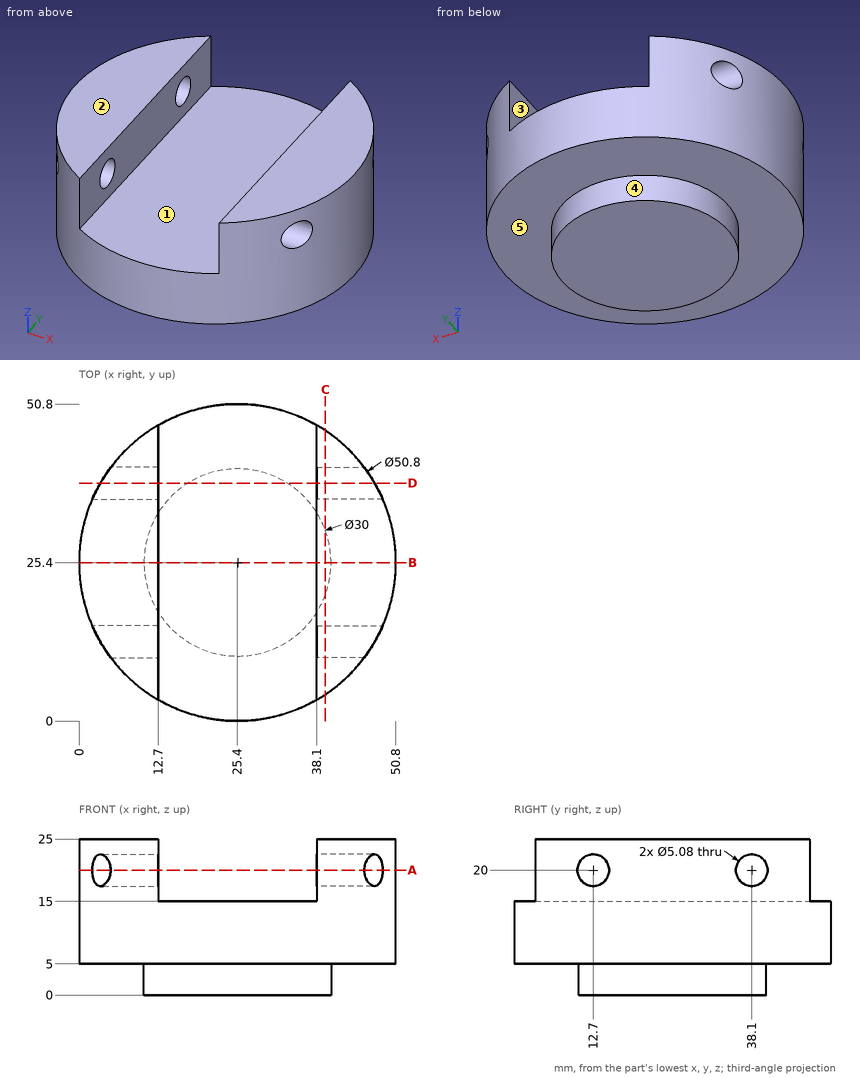
The figure shows three views and two pictorial views of one solid part (mm, origin at its lowest corner). Answer the questions. A direction names the side the tool comes from. Round coordinates to 2 decimals unless told otherwise and drop trailing zeros. Write each loop counter-clockwise with the first axis right and the second up, starting at its lowest first coordinate (ties: lowest second). Pieces come first, ordered by that corner, then holes. Notation, with made-up numbers: (34, 38) -> (40, 38) arc R22 cw to (40, 53) -> close; hole circle Ø5 at (-7.5, -11.5). An arc over 180 degrees is marked (long way). Write each question's results on one line, items separated by ' | '.
Q1. Section D-D, the plane y = 38.1 is taken. Write down the section's boundary in (x, z), then the cut area to 3 significant figures.
Data:
outline: (3.4, 5) -> (17.42, 5) -> (17.42, 0) -> (33.38, 0) -> (33.38, 5) -> (47.4, 5) -> (47.4, 17.46) -> (38.1, 17.46) -> (38.1, 15) -> (12.7, 15) -> (12.7, 17.46) -> (3.4, 17.46) -> close; (3.4, 22.54) -> (12.7, 22.54) -> (12.7, 25) -> (3.4, 25) -> close; (38.1, 22.54) -> (47.4, 22.54) -> (47.4, 25) -> (38.1, 25) -> close | area: 611 mm^2
Q2. Flat-ended cylindrical pins translate along their axes: P1, Ø12, axis at x = 28.5, y = 6, coming from the +Z side; P2, Ø8, axis at y = 38.1, z = 20, coming from the +X side; P3, Ø5, axis at x = 8.5, y = 38.5, coming from the -Z side. Find the tip coordinate at first contact, or state that the pin passes through.
Data:
P1: z = 15 | P2: x = 49.26 | P3: z = 5
Q3. Straight lines are drawn through the part: line 1 along Z through (x, y) = (42.5, 12.7); line 2 along Y through (x, z) = (7.25, 20); line 3 along Y through (x, z) = (42.75, 20). For each, find the intervals that lie inside material, in ascending order. Write a range as [from, to].
Data:
line 1: [5, 17.46], [22.54, 25] | line 2: [7.63, 10.16], [15.24, 35.56], [40.64, 43.17] | line 3: [6.85, 10.16], [15.24, 35.56], [40.64, 43.95]
Q4. Determine the mould class of the marked faces 3, 4 and 5 for opening direction X: released by +X, released by -X, zero draft, split by the parting line, or undercut.
Data:
face 3: undercut | face 4: split by the parting line | face 5: zero draft
Q5. Section C-C, the plane x = 39.5 is taken. Write down the section's boundary in (y, z).
Data:
outline: (4.27, 5) -> (20.28, 5) -> (20.28, 0) -> (30.52, 0) -> (30.52, 5) -> (46.53, 5) -> (46.53, 25) -> (4.27, 25) -> close; hole circle Ø5.08 at (12.7, 20); hole circle Ø5.08 at (38.1, 20)
Q6. Section A-A, the plane z = 20 is taken. Write down the section's boundary in (x, y).
Data:
outline: (2.12, 15.24) -> (12.7, 15.24) -> (12.7, 35.56) -> (2.12, 35.56) arc R25.4 ccw to start; (5.08, 10.16) arc R25.4 ccw to (12.7, 3.4) -> (12.7, 10.16) -> close; (5.08, 40.64) -> (12.7, 40.64) -> (12.7, 47.4) arc R25.4 ccw to start; (38.1, 3.4) arc R25.4 ccw to (45.72, 10.16) -> (38.1, 10.16) -> close; (38.1, 15.24) -> (48.68, 15.24) arc R25.4 ccw to (48.68, 35.56) -> (38.1, 35.56) -> close; (38.1, 40.64) -> (45.72, 40.64) arc R25.4 ccw to (38.1, 47.4) -> close
Q7. Section B-B, the plane y = 25.4 is taken. Write down the section's boundary in (x, z).
Data:
outline: (0, 5) -> (10.4, 5) -> (10.4, 0) -> (40.4, 0) -> (40.4, 5) -> (50.8, 5) -> (50.8, 25) -> (38.1, 25) -> (38.1, 15) -> (12.7, 15) -> (12.7, 25) -> (0, 25) -> close
Q8. Which of the six approach directions +Z, -Z, +X, -X, +Y, -Y give full straight-line access (tool end or side, diameter ignored) to the marked faces 1 and 2?
Data:
face 1: +Z, +Y, -Y | face 2: +Z, +X, -X, +Y, -Y
